Study the drawing (mm; zero at the part's minimum x, y, z) and answer. A direction names the side the tool comes from. Give positions to 0.01 mm unless a question says otherwise; leave off trailing zeros. Write each loop counter-clockwise with the first axis right and the second up, starting at its lowest first coordinate (ties: lowest second). Pieces come first, ordered by that corner, then holes. Notation, with made-up numbers: M -30,58 L -12,58 A37 ccw -12,97 Z; hole C 9,81 d3. An arc over 180 degrees is marked long. Use a Markdown table: item, result. Add a question column.
Item 1: A cutting plane is placed at B-B on x = 18.75. Determine the outline of the cut face in (y, z), then the cut area to 3 significant figures.
Item 2: A cutting plane is placed at A-A on z = 38.5. Determine the outline of the cut face in (x, y).
Item 3: The mould has two halves that part along X. Classify the marked faces 1, 2 and 3: pulls with the +X half, pulls with the -X half, needs draft (parallel to the pull), parting line crosses it, or undercut.
Item 4: Given P1, Ø1.8, axis at x = 19, z = 48, coming from the +Y side; P2, Ø3, axis at x = 18.5, y = 18.5, coming from the -Z side; P3, Ø1.6, axis at x = 9, z = 27.5, coming from the +Y side, each flat-ended and moving along its own axis, determine where each tip first touches the part or whether it passes through.
Item 5: A cutting plane is placed at C-C on y = 8. Determine the outline of the cut face in (x, z), then the cut area to 3 significant figures.
Item 6: For the marked faces 4, 5, 6 and 7, determine the directions among +Z, -Z, +X, -X, +Y, -Y from which every point of the face is accessible in a straight line to the end or side of a thin tool.
Item 7: A cutting plane is placed at D-D on z = 23. Determine the outline of the cut face in (x, y).
Item 8: Consider probe 1 along Z at (x, y) = (19.5, 9.5); probe 2 along X at (y, z) = (7.25, 31.5); probe 3 along Z at (x, y) = (18.5, 6.25). Determine where each line is inside the solid, lowest interval first. Write a range as [from, to].
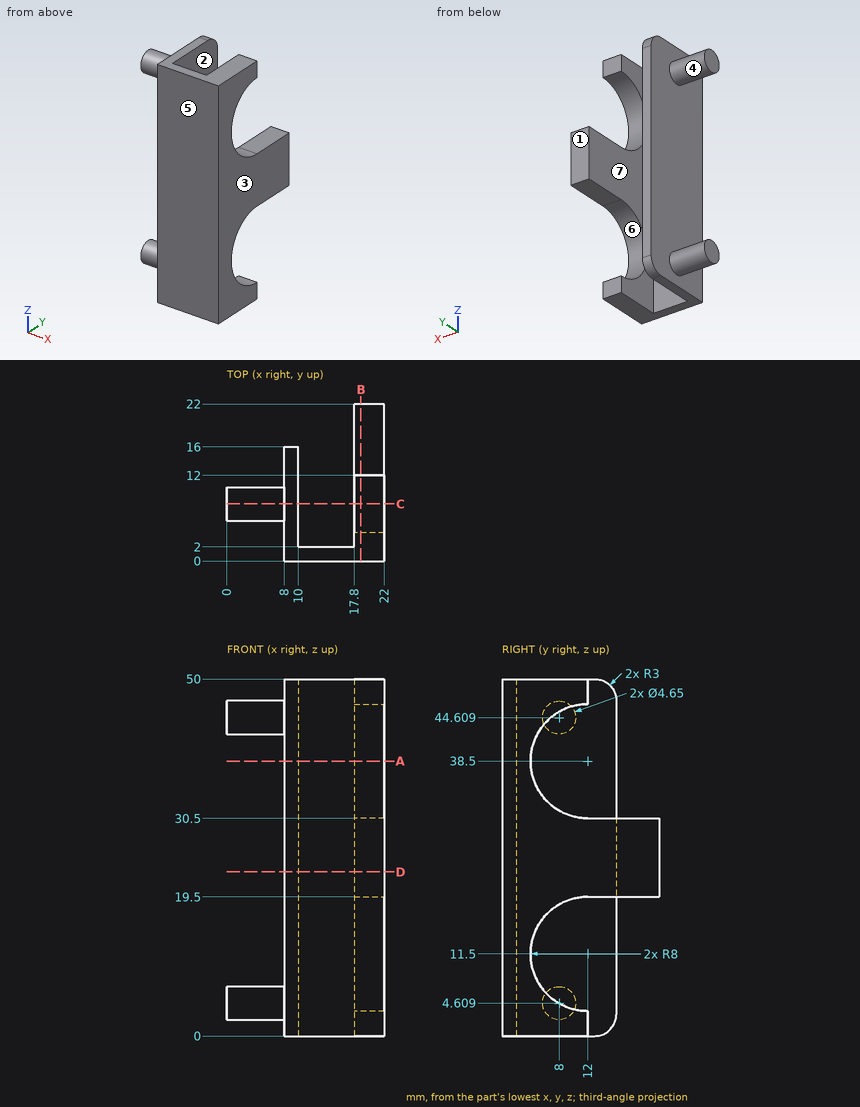
Filled in:
| question | item | result |
|---|---|---|
| 1 | outline | M 0,0 L 12,0 L 12,3.5 A8 cw 12,19.5 L 22,19.5 L 22,30.5 L 12,30.5 A8 cw 12,46.5 L 12,50 L 0,50 Z |
| 1 | area | 509 mm² |
| 2 | outline | M 8,0 L 22,0 L 22,4 L 17.8,4 L 17.8,2 L 10,2 L 10,16 L 8,16 Z |
| 3 | face 1 | needs draft |
| 3 | face 2 | undercut |
| 3 | face 3 | pulls with the +X half |
| 4 | P1 | y = 12 |
| 4 | P2 | z = 19.5 |
| 4 | P3 | y = 16 |
| 5 | outline | M 0,2.28 L 8,2.28 L 8,0 L 10,0 L 10,50 L 8,50 L 8,46.93 L 0,46.93 L 0,42.28 L 8,42.28 L 8,6.93 L 0,6.93 Z; M 17.8,0 L 22,0 L 22,4.57 L 17.8,4.57 Z; M 17.8,18.43 L 22,18.43 L 22,31.57 L 17.8,31.57 Z; M 17.8,45.43 L 22,45.43 L 22,50 L 17.8,50 Z |
| 5 | area | 268 mm² |
| 6 | face 4 | -X |
| 6 | face 5 | +Z, -Z, +X, -X, -Y |
| 6 | face 6 | +X, +Y |
| 6 | face 7 | +Z, -Z, +Y |
| 7 | outline | M 8,0 L 22,0 L 22,22 L 17.8,22 L 17.8,2 L 10,2 L 10,16 L 8,16 Z |
| 8 | probe 1 | [0, 3.9], [19.1, 30.9], [46.1, 50] |
| 8 | probe 2 | [8, 10], [17.8, 22] |
| 8 | probe 3 | [0, 5.94], [17.06, 32.94], [44.06, 50] |
